from build123d import *

# Parameters (mm, degrees)
BOSS_EXTRUDE1_DEPTH = 8.128
CUT_EXTRUDE1_DEPTH  = 0.254
FILLET3_R           = 1.27
SHELL2_T            = -0.508
SKETCH4_R           = 16.002
SKETCH4_R_2         = 6.35
CUT_EXTRUDE3_DEPTH  = 8.874
SKETCH6_R           = 7.62
SKETCH6_R_2         = 6.35
BOSS_EXTRUDE5_DEPTH = 0.508


with BuildPart() as part:
    # Sketch1 → Boss-Extrude1 (new body)
    with BuildSketch(Plane.XY):
        with BuildLine():
            Line((34.735008, -51.816), (-34.735008, -51.816))
            ThreePointArc((-34.735008, -51.816), (-37.563429468, -50.644429468), (-38.735, -47.816008))
            Line((-38.735, -47.816008), (-38.735, 47.816008))
            ThreePointArc((-38.735, 47.816008), (-37.563429468, 50.644429468), (-34.735008, 51.816))
            Line((-34.735008, 51.816), (34.735008, 51.816))
            ThreePointArc((34.735008, 51.816), (37.563429468, 50.644429468), (38.735, 47.816008))
            Line((38.735, 47.816008), (38.735, -47.816008))
            ThreePointArc((38.735, -47.816008), (37.563429468, -50.644429468), (34.735008, -51.816))
        make_face()
    extrude(amount=-BOSS_EXTRUDE1_DEPTH)

    # Sketch3 → Cut-Extrude1 (cut)
    with BuildSketch(Plane.XY):
        with BuildLine():
            Line((-28.385008, -44.45), (28.385008, -44.45))
            ThreePointArc((28.385008, -44.45), (31.213429468, -43.278429468), (32.385, -40.450008))
            Line((32.385, -40.450008), (32.385, 40.450008))
            ThreePointArc((32.385, 40.450008), (31.213429468, 43.278429468), (28.385008, 44.45))
            Line((28.385008, 44.45), (-28.385008, 44.45))
            ThreePointArc((-28.385008, 44.45), (-31.213429468, 43.278429468), (-32.385, 40.450008))
            Line((-32.385, 40.450008), (-32.385, -40.450008))
            ThreePointArc((-32.385, -40.450008), (-31.213429468, -43.278429468), (-28.385008, -44.45))
        make_face()
    extrude(amount=-CUT_EXTRUDE1_DEPTH, mode=Mode.SUBTRACT)

    # Fillet3
    fillet3_edges = [part.edges().sort_by_distance(p)[0] for p in [
        (38.735, 0, 0),
        (37.563429468, -50.644429468, 0),
        (0, -51.816, 0),
        (-37.563429468, -50.644429468, 0),
        (-38.735, 0, 0),
        (-37.563429468, 50.644429468, 0),
        (0, 51.816, 0),
        (37.563429468, 50.644429468, 0),
    ]]
    fillet(fillet3_edges, radius=FILLET3_R)

    # Shell2
    shell2_openings = [part.faces().sort_by_distance(p)[0] for p in [
        (0, 0, -8.128),
    ]]
    offset(amount=SHELL2_T, openings=shell2_openings, kind=Kind.INTERSECTION)

    # Sketch4 → Cut-Extrude3 (cut, through all)
    with BuildSketch(Plane.XY.offset(-0.254)):
        with Locations((0, 0.254)):
            Circle(SKETCH4_R)
        with Locations((17.907, 34.036)):
            Circle(SKETCH4_R_2)
        with Locations((-17.907, 34.036)):
            Circle(SKETCH4_R_2)
    extrude(amount=-CUT_EXTRUDE3_DEPTH, mode=Mode.SUBTRACT)

    # Sketch6 → Boss-Extrude5 (add)
    with BuildSketch(Plane.XY.offset(-0.254)):
        with Locations((-17.907, 34.036)):
            Circle(SKETCH6_R)
        with Locations((-17.907, 34.036)):
            Circle(SKETCH6_R_2, mode=Mode.SUBTRACT)
        with Locations((17.907, 34.036)):
            Circle(SKETCH6_R)
        with Locations((17.907, 34.036)):
            Circle(SKETCH6_R_2, mode=Mode.SUBTRACT)
    extrude(amount=BOSS_EXTRUDE5_DEPTH)


solid = part.part
Design review of the part built by this model. Coordinates are the model's own, in mm. A direction names the side the tool comes from. Coordinates: 2 decimals unless noted, no trailing zeros. Loops run counter-clockwise (first coordinate to the right, second up) from the corner with the lowest first, then second, coordinate; pieces in that order, holes last.
Item 1: For faces 1 (the cylindrical face through (37.23, -50.26, -4.65)), 2 (the cylindrical face through (37.594, -50.613, -4.651)), 3 (the cylindrical face through (25.175, 36.325, -0.004)), list the 3-axis set-ups (+Z, -Z, +X, -X, +Y, -Y) from which the entire face can be reached by the end or side of a thin tool; tool diameter is ignored.
Completed:
face 1: -Z
face 2: +Z, -Z, +X, -Y
face 3: +Z
Item 2: Add section D-D (x = 29.5). Write out the cut boundary in (y, z).
Completed:
outline: (-51.82, -8.13) - (-51.31, -8.13) - (-51.31, -1.27) arc R0.76 cw to (-50.55, -0.51) - (-44.82, -0.51) - (-44.82, -0.76) - (44.82, -0.76) - (44.82, -0.51) - (50.55, -0.51) arc R0.76 cw to (51.31, -1.27) - (51.31, -8.13) - (51.82, -8.13) - (51.82, -1.27) arc R1.27 ccw to (50.55, 0) - (44.29, 0) - (44.29, -0.25) - (-44.29, -0.25) - (-44.29, 0) - (-50.55, 0) arc R1.27 ccw to (-51.82, -1.27) - close
Item 3: Clearance check with flat-ended pins moving along their axes: pin 1 (16.5 mm diameter, centred on x = 17.907, y = 34.036, fed in from +Z); pin 2 (2 mm diameter, centred on x = -27, y = -25, fed in from -Z). State where each tip first meets the part, or that it passes through.
Completed:
pin 1: stops at z = 0.25
pin 2: stops at z = -0.76
Item 4: Add section A-A (x = 0). Write out the cut boundary in (y, z).
Completed:
outline: (-51.82, -8.13) - (-51.31, -8.13) - (-51.31, -1.27) arc R0.76 cw to (-50.55, -0.51) - (-44.96, -0.51) - (-44.96, -0.76) - (-15.75, -0.76) - (-15.75, -0.25) - (-44.45, -0.25) - (-44.45, 0) - (-50.55, 0) arc R1.27 ccw to (-51.82, -1.27) - close; (16.26, -0.76) - (44.96, -0.76) - (44.96, -0.51) - (50.55, -0.51) arc R0.76 cw to (51.31, -1.27) - (51.31, -8.13) - (51.82, -8.13) - (51.82, -1.27) arc R1.27 ccw to (50.55, 0) - (44.45, 0) - (44.45, -0.25) - (16.26, -0.25) - close
Item 5: Add section C-C (x = 20). Write out the cut boundary in (y, z).
Completed:
outline: (-51.82, -8.13) - (-51.31, -8.13) - (-51.31, -1.27) arc R0.76 cw to (-50.55, -0.51) - (-44.96, -0.51) - (-44.96, -0.76) - (28.04, -0.76) - (28.04, 0.25) - (26.71, 0.25) - (26.71, -0.25) - (-44.45, -0.25) - (-44.45, 0) - (-50.55, 0) arc R1.27 ccw to (-51.82, -1.27) - close; (40.03, -0.76) - (44.96, -0.76) - (44.96, -0.51) - (50.55, -0.51) arc R0.76 cw to (51.31, -1.27) - (51.31, -8.13) - (51.82, -8.13) - (51.82, -1.27) arc R1.27 ccw to (50.55, 0) - (44.45, 0) - (44.45, -0.25) - (41.36, -0.25) - (41.36, 0.25) - (40.03, 0.25) - close
Item 6: Add section B-B (z = -5). Write out the cut boundary in (x, y) (3 decimals).
Completed:
outline: (-38.735, -47.816) arc R4 ccw to (-34.735, -51.816) - (34.735, -51.816) arc R4 ccw to (38.735, -47.816) - (38.735, 47.816) arc R4 ccw to (34.735, 51.816) - (-34.735, 51.816) arc R4 ccw to (-38.735, 47.816) - close; hole (-38.227, -47.816) arc R3.492 ccw to (-34.735, -51.308) - (34.735, -51.308) arc R3.492 ccw to (38.227, -47.816) - (38.227, 47.816) arc R3.492 ccw to (34.735, 51.308) - (-34.735, 51.308) arc R3.492 ccw to (-38.227, 47.816) - close
Item 7: Wall thickness on L1, parallel to Y at x = -33.5, z = -3.5; L2, parallel to X at y = 10.5, z = -7 (3 decimals); L3, parallel to Z at x = 11, y = 41.5: over which ranges is each line inside the solid? List them lowest first.
Completed:
L1: y = -51.82 to -51.31, 51.31 to 51.82
L2: x = -38.735 to -38.227, 38.227 to 38.735
L3: z = -0.76 to -0.25
